Geometry check sheet. Reference: the model listing, model coordinates, mm. A direction names the side the tool comes from. Coordinates: 2 decimals unless noted, no trailing zeros. Write each loop counter-clockwise with the first axis right and the second up, starting at its lowest first coordinate (ties: lowest second). Pieces come first, ordered by that corner, then holes. Notation, with made-up numbers: (81.25, 12.25) -> (96.25, 12.25) arc R5 cw to (96.25, 16.25) -> close; hole circle Ø11 at (85, 70). An arc over 180 degrees is marked (long way). Answer in a Markdown table with one row per item. Add a question column.
1. Mould release check, pull along X, two halves, no side actions. Record for faces 5 (the cylindrical face through (-32.517, 646.433, -479.083)), 6 (the cylindrical face through (-17.57, 742.48, -1083.85)), 7 (the flat face through (56.3, 800, -1072.9)): pulls with the +X half, pulls with the -X half, needs draft (parallel to the pull), parting line crosses it, or undercut.
2. Cross-section at D-D on x = 55.5. Record the cut outline in (y, z).
3. Depth check by flat-ended pin: P1, Ø3, axis at y = 612.5, z = -219.5, coming from the +X side; P2, Ø1.5, axis at x = -74.5, z = -677.5, coming from the -Y side; P3, Ø8, axis at y = 549, z = -510.5, coming from the -X side. Enter the tip coordinate at first touch or a pass-through.
4. Cross-section at C-C on y = 71. Record the cut outline in (x, z).
5. Scan lines: L1, parallel to Z at x = 0, y = 766; L2, parallel to X at y = 136.5, z = 0; L3, parallel to Y at x = 0, z = -537. Record each from-to range of solid material in increasing order. Write a range as from..to.
6. Cross-section at B-B on z = -296. Record the cut outline in (x, y), and give its area (3 significant figures).
7. Set-up check for faces 1 (the cylindrical face through (-29.27, 631.79, -479.08)), 2 (the cylindrical face through (80.64, 742.48, -1076.48)), 3 (the flat face through (56.3, 0, -122.9)), 4 (the cylindrical face through (-19.527, 160.552, -148.724)): record each of +Z, -Z, +X, -X, +Y, -Y from which the full face is reachable in a straight line by a thin tool's end or side.
8. Cross-section at A-A on x = 0. Record the cut outline in (y, z), and give its area (3 significant figures).
```python
from build123d import *

# Parameters (mm, degrees)
SKETCH2_R   = 150
SKETCH2_R_2 = 135


with BuildPart() as part:
    # Sweep2: sweep along a path in Sketch1
    with BuildLine(Plane(origin=(0, 0, 0), x_dir=(0, 0, -1), z_dir=(1, 0, 0))) as sweep2_path:
        Line((0, 0), (0, 316.67))
        ThreePointArc((0, 316.67), (53.696113805, 446.303886195), (183.33, 500))
        Line((183.33, 500), (500, 500))
        Line((500, 500), (766.67, 500))
        ThreePointArc((766.67, 500), (896.303886195, 553.696113805), (950, 683.33))
        Line((950, 683.33), (950, 800))
    # Sketch2 → Sweep2 (sweep)
    with BuildSketch(Plane(origin=(0, 0, 0), x_dir=(1, 0, 0), z_dir=(0, 1, 0))):
        Circle(SKETCH2_R)
        Circle(SKETCH2_R_2, mode=Mode.SUBTRACT)
    sweep(path=sweep2_path.line)


solid = part.part
```
Results found:
| question | item | result |
|---|---|---|
| 1 | face 5 | parting line crosses it |
| 1 | face 6 | undercut |
| 1 | face 7 | needs draft |
| 2 | outline | (0, -139.35) -> (316.67, -139.35) arc R43.98 cw to (360.65, -183.33) -> (360.65, -766.67) arc R322.68 ccw to (683.33, -1089.35) -> (800, -1089.35) -> (800, -1073.06) -> (683.33, -1073.06) arc R306.39 cw to (376.94, -766.67) -> (376.94, -183.33) arc R60.27 ccw to (316.67, -123.06) -> (0, -123.06) -> close; (0, 123.06) -> (316.67, 123.06) arc R306.39 cw to (623.06, -183.33) -> (623.06, -766.67) arc R60.27 ccw to (683.33, -826.94) -> (800, -826.94) -> (800, -810.65) -> (683.33, -810.65) arc R43.98 cw to (639.35, -766.67) -> (639.35, -183.33) arc R322.68 ccw to (316.67, 139.35) -> (0, 139.35) -> close |
| 3 | P1 | stops at x = 100.89 |
| 3 | P2 | stops at y = 369.38 |
| 3 | P3 | stops at x = -143.09 |
| 4 | outline | circle Ø300 at (0, 0); hole circle Ø270 at (0, 0) |
| 5 | L1 | z = -1100..-1085, -815..-800 |
| 5 | L2 | x = -150..-135, 135..150 |
| 5 | L3 | y = 350..365, 635..650 |
| 6 | outline | circle Ø300 at (0, 500); hole circle Ø270 at (0, 500) |
| 6 | area | 13,400 mm^2 |
| 7 | face 1 | none |
| 7 | face 2 | +Y |
| 7 | face 3 | +Z, -Z, +X, -X, -Y |
| 7 | face 4 | -Y |
| 8 | outline | (0, -150) -> (316.67, -150) arc R33.33 cw to (350, -183.33) -> (350, -766.67) arc R333.33 ccw to (683.33, -1100) -> (800, -1100) -> (800, -1085) -> (683.33, -1085) arc R318.33 cw to (365, -766.67) -> (365, -183.33) arc R48.33 ccw to (316.67, -135) -> (0, -135) -> close; (0, 135) -> (316.67, 135) arc R318.33 cw to (635, -183.33) -> (635, -766.67) arc R48.33 ccw to (683.33, -815) -> (800, -815) -> (800, -800) -> (683.33, -800) arc R33.33 cw to (650, -766.67) -> (650, -183.33) arc R333.33 ccw to (316.67, 150) -> (0, 150) -> close |
| 8 | area | 47,800 mm^2 |
